```python
from build123d import *

# Parameters (mm, degrees)
BOSS_EXTRUDE1_DEPTH = 34
SKETCH7_W           = 4
SKETCH7_H           = 8
BOSS_EXTRUDE3_DEPTH = 10
SKETCH9_R           = 1.51
CUT_EXTRUDE5_DEPTH  = 48.193431746
FILLET2_R           = 4
SKETCH16_R          = 1.5
CUT_EXTRUDE7_DEPTH  = 30
CHAMFER1_SIZE       = 2


# Some blends are built 0.0001 mm under size
with BuildPart() as part:
    # Sketch1 → Boss-Extrude1 (new body)
    with BuildSketch(Plane(origin=(0, 0, 0), x_dir=(1, 0, 0), z_dir=(0, 1, 0))):
        with BuildLine():
            Line((-7.9, 5.966573556), (-7.9, -5.966573556))
            ThreePointArc((-7.9, -5.966573556), (0, -9.9), (7.9, -5.966573556))
            Line((7.9, -5.966573556), (7.9, 5.966573556))
            ThreePointArc((7.9, 5.966573556), (0, 9.9), (-7.9, 5.966573556))
        make_face()
    extrude(amount=BOSS_EXTRUDE1_DEPTH)

    # Sketch7 → Boss-Extrude3 (add)
    with BuildSketch(Plane(origin=(0, 34, 0), x_dir=(1, 0, 0), z_dir=(0, 1, 0))):
        with Locations((-4, 0)):
            Rectangle(SKETCH7_W, SKETCH7_H)
        with Locations((4, 0)):
            Rectangle(SKETCH7_W, SKETCH7_H)
    extrude(amount=BOSS_EXTRUDE3_DEPTH)

    # Sketch9 → Cut-Extrude5 (cut, through all)
    with BuildSketch(Plane(origin=(6, 0, 0), x_dir=(0, 0, -1), z_dir=(1, 0, 0))):
        with Locations((0, 40)):
            Circle(SKETCH9_R)
    extrude(amount=-CUT_EXTRUDE5_DEPTH, mode=Mode.SUBTRACT)

    # Fillet2
    fillet2_edges = [part.edges().sort_by_distance(p)[0] for p in [
        (4, 44, 4),
        (4, 44, -4),
        (-4, 44, -4),
        (-4, 44, 4),
    ]]
    fillet(fillet2_edges, radius=FILLET2_R - 0.0001)  # a hair under: the kernel refuses the full size

    # Sketch16 → Cut-Extrude7 (cut)
    with BuildSketch(Plane.XZ):
        with Locations(Location((0, 0, 0), (0, 0, 270))):
            Circle(SKETCH16_R)
    extrude(amount=-CUT_EXTRUDE7_DEPTH, mode=Mode.SUBTRACT)

    # Chamfer1
    # the kernel refuses this chamfer: 2 mm, written as the material it adds along each edge
    with BuildSketch(Plane(origin=(-6, 34, -4), x_dir=(0, -0.027495876610585623, -0.9996219169112968), z_dir=(1, 0, 0)), Plane(origin=(2, 34, -4), x_dir=(0, -0.027495876610585623, -0.9996219169112968), z_dir=(1, 0, 0)), Plane(origin=(6, 34, 4), x_dir=(0, -0.027495876610585623, 0.9996219169112968), z_dir=(-1, 0, 0))) as chamfer1_piece_1:
        Polygon((CHAMFER1_SIZE * 0.999621916911, CHAMFER1_SIZE * 0.0274958766106), (-CHAMFER1_SIZE * 0.0274958766106, CHAMFER1_SIZE * 0.999621916911), (0, 0), align=None)
    extrude(amount=4)
    with BuildSketch(Plane(origin=(-6, 34, -4), x_dir=(0, -0.027495876610585623, -0.9996219169112968), z_dir=(1, 0, 0))) as chamfer1_piece_2_section:
        Polygon((CHAMFER1_SIZE * 0.999621916911, CHAMFER1_SIZE * 0.0274958766106), (-CHAMFER1_SIZE * 0.0274958766106, CHAMFER1_SIZE * 0.999621916911), (0, 0), align=None)
    chamfer1_piece_2 = extrude(amount=9.143365976, mode=Mode.PRIVATE)
    chamfer1_piece_2 = split(chamfer1_piece_2, bisect_by=Plane(origin=(2, 34.659587254, -4.659587254), z_dir=(1, 0, 0)), keep=Keep.TOP, mode=Mode.PRIVATE)
    add(chamfer1_piece_2)
    with BuildSketch(Plane(origin=(-6, 34, 4), x_dir=(0.02749587661058651, 0.9996219169112968, 0), z_dir=(0, 0, -1))) as chamfer1_piece_3_section:
        Polygon((CHAMFER1_SIZE * 0.999621916911, -CHAMFER1_SIZE * 0.0274958766106), (-CHAMFER1_SIZE * 0.0274958766106, -CHAMFER1_SIZE * 0.999621916911), (0, 0), align=None)
    chamfer1_piece_3 = extrude(amount=8, mode=Mode.PRIVATE)
    chamfer1_piece_3 = split(chamfer1_piece_3, bisect_by=Plane(origin=(-7.9, 34.66508919, 0), z_dir=(1, 0, 0)), keep=Keep.TOP, mode=Mode.PRIVATE)
    add(chamfer1_piece_3)
    with BuildSketch(Plane(origin=(3.143365976, 34, 4), x_dir=(0, 0.9996219169112968, -0.027495876610586296), z_dir=(-1, 0, 0))) as chamfer1_piece_4_section:
        Polygon((CHAMFER1_SIZE * 0.999621916911, -CHAMFER1_SIZE * 0.0274958766106), (-CHAMFER1_SIZE * 0.0274958766106, -CHAMFER1_SIZE * 0.999621916911), (0, 0), align=None)
    chamfer1_piece_4 = extrude(amount=9.143365976, mode=Mode.PRIVATE)
    chamfer1_piece_4 = split(chamfer1_piece_4, bisect_by=Plane(origin=(2, 34.659587254, 4.659587254), z_dir=(1, 0, 0)), keep=Keep.TOP, mode=Mode.PRIVATE)
    add(chamfer1_piece_4)
    with BuildSketch(Plane(origin=(-2, 34, 4), x_dir=(0, 0.9996219169112968, -0.027495876610586296), z_dir=(-1, 0, 0))) as chamfer1_piece_5:
        Polygon((CHAMFER1_SIZE * 0.999621916911, -CHAMFER1_SIZE * 0.0274958766106), (-CHAMFER1_SIZE * 0.0274958766106, -CHAMFER1_SIZE * 0.999621916911), (0, 0), align=None)
    extrude(amount=4)
    with BuildSketch(Plane(origin=(-3.143365976, 34, -4), x_dir=(0, -0.027495876610585623, -0.9996219169112968), z_dir=(1, 0, 0))) as chamfer1_piece_6_section:
        Polygon((CHAMFER1_SIZE * 0.999621916911, CHAMFER1_SIZE * 0.0274958766106), (-CHAMFER1_SIZE * 0.0274958766106, CHAMFER1_SIZE * 0.999621916911), (0, 0), align=None)
    chamfer1_piece_6 = extrude(amount=9.143365976, mode=Mode.PRIVATE)
    chamfer1_piece_6 = split(chamfer1_piece_6, bisect_by=Plane(origin=(-2, 34.659587254, -4.659587254), z_dir=(-1, 0, 0)), keep=Keep.TOP, mode=Mode.PRIVATE)
    add(chamfer1_piece_6)
    with BuildSketch(Plane(origin=(6, 34, 4), x_dir=(0, -0.027495876610585623, 0.9996219169112968), z_dir=(-1, 0, 0))) as chamfer1_piece_7_section:
        Polygon((CHAMFER1_SIZE * 0.999621916911, CHAMFER1_SIZE * 0.0274958766106), (-CHAMFER1_SIZE * 0.0274958766106, CHAMFER1_SIZE * 0.999621916911), (0, 0), align=None)
    chamfer1_piece_7 = extrude(amount=9.143365976, mode=Mode.PRIVATE)
    chamfer1_piece_7 = split(chamfer1_piece_7, bisect_by=Plane(origin=(-2, 34.659587254, 4.659587254), z_dir=(-1, 0, 0)), keep=Keep.TOP, mode=Mode.PRIVATE)
    add(chamfer1_piece_7)
    with BuildSketch(Plane(origin=(6, 34, -4), x_dir=(0.9996219169112968, -0.027495876610585623, 0), z_dir=(0, 0, 1))) as chamfer1_piece_8_section:
        Polygon((CHAMFER1_SIZE * 0.999621916911, CHAMFER1_SIZE * 0.0274958766106), (-CHAMFER1_SIZE * 0.0274958766106, CHAMFER1_SIZE * 0.999621916911), (0, 0), align=None)
    chamfer1_piece_8 = extrude(amount=8, mode=Mode.PRIVATE)
    chamfer1_piece_8 = split(chamfer1_piece_8, bisect_by=Plane(origin=(7.9, 34.66508919, 0), z_dir=(-1, 0, 0)), keep=Keep.TOP, mode=Mode.PRIVATE)
    add(chamfer1_piece_8)
    with BuildSketch(Plane(origin=(-6, 34, 4), x_dir=(0.02749587661058651, 0.9996219169112968, 0), z_dir=(0, 0, -1))) as chamfer1_piece_9a_section:
        Polygon((CHAMFER1_SIZE * 0.999621916911, -CHAMFER1_SIZE * 0.0274958766106), (-CHAMFER1_SIZE * 0.0274958766106, -CHAMFER1_SIZE * 0.999621916911), (0, 0), align=None)
    chamfer1_piece_9a = extrude(amount=13.143365976, mode=Mode.PRIVATE)
    chamfer1_piece_9a = split(chamfer1_piece_9a, bisect_by=Plane(origin=(-6.579477658, 34.702229701, -4), z_dir=(0, 0, -1)), keep=Keep.TOP, mode=Mode.PRIVATE)
    chamfer1_piece_9a = chamfer1_piece_9a & Plane(origin=(0, 34.702229701, 0), x_dir=(-0.7979797979797981, 0, 0.6026841975828805), z_dir=(0, -1, 0)) * Cylinder(9.9, 35, mode=Mode.PRIVATE)
    chamfer1_piece_9a = split(chamfer1_piece_9a, bisect_by=Plane(origin=(-7.9, 34.702229701, -5.684853753), z_dir=(1, 0, 0)), keep=Keep.TOP, mode=Mode.PRIVATE)
    with BuildSketch(Plane(origin=(-11.143365976, 34, -4), x_dir=(0, -0.027495876610585623, -0.9996219169112968), z_dir=(1, 0, 0))) as chamfer1_piece_9b_section:
        Polygon((CHAMFER1_SIZE * 0.999621916911, CHAMFER1_SIZE * 0.0274958766106), (-CHAMFER1_SIZE * 0.0274958766106, CHAMFER1_SIZE * 0.999621916911), (0, 0), align=None)
    chamfer1_piece_9b = extrude(amount=9.143365976, mode=Mode.PRIVATE)
    chamfer1_piece_9b = split(chamfer1_piece_9b, bisect_by=Plane(origin=(-6, 34.659622918, -4.659519528), z_dir=(-1, 0, 0)), keep=Keep.TOP, mode=Mode.PRIVATE)
    chamfer1_piece_9b = split(chamfer1_piece_9b, bisect_by=Plane(origin=(-7.9, 34.659622918, -4.659519528), z_dir=(1, 0, 0)), keep=Keep.TOP, mode=Mode.PRIVATE)
    chamfer1_piece_9b = chamfer1_piece_9b & Plane(origin=(0, 34.659622918, 0), x_dir=(0.7979797979797981, 0, -0.6026841975828805), z_dir=(0, -1, 0)) * Cylinder(9.9, 27, mode=Mode.PRIVATE)
    chamfer1_piece_9 = chamfer1_piece_9a & chamfer1_piece_9b
    add(chamfer1_piece_9)
    with BuildSketch(Plane(origin=(-6, 34, 9.143365976), x_dir=(0.02749587661058651, 0.9996219169112968, 0), z_dir=(0, 0, -1))) as chamfer1_piece_10a_section:
        Polygon((CHAMFER1_SIZE * 0.999621916911, -CHAMFER1_SIZE * 0.0274958766106), (-CHAMFER1_SIZE * 0.0274958766106, -CHAMFER1_SIZE * 0.999621916911), (0, 0), align=None)
    chamfer1_piece_10a = extrude(amount=13.143365976, mode=Mode.PRIVATE)
    chamfer1_piece_10a = split(chamfer1_piece_10a, bisect_by=Plane(origin=(-6.579477657, 34.702229707, 4), z_dir=(0, 0, 1)), keep=Keep.TOP, mode=Mode.PRIVATE)
    chamfer1_piece_10a = chamfer1_piece_10a & Plane(origin=(0, 34.702229707, 0), x_dir=(-0.7979797979797981, 0, 0.6026841975828805), z_dir=(0, -1, 0)) * Cylinder(9.9, 35, mode=Mode.PRIVATE)
    chamfer1_piece_10a = split(chamfer1_piece_10a, bisect_by=Plane(origin=(-7.9, 34.702229707, 5.684853748), z_dir=(1, 0, 0)), keep=Keep.TOP, mode=Mode.PRIVATE)
    with BuildSketch(Plane(origin=(-2, 34, 4), x_dir=(0, 0.9996219169112968, -0.027495876610586296), z_dir=(-1, 0, 0))) as chamfer1_piece_10b_section:
        Polygon((CHAMFER1_SIZE * 0.999621916911, -CHAMFER1_SIZE * 0.0274958766106), (-CHAMFER1_SIZE * 0.0274958766106, -CHAMFER1_SIZE * 0.999621916911), (0, 0), align=None)
    chamfer1_piece_10b = extrude(amount=9.143365976, mode=Mode.PRIVATE)
    chamfer1_piece_10b = split(chamfer1_piece_10b, bisect_by=Plane(origin=(-6, 34.659622918, 4.659519528), z_dir=(-1, 0, 0)), keep=Keep.TOP, mode=Mode.PRIVATE)
    chamfer1_piece_10b = chamfer1_piece_10b & Plane(origin=(0, 34.659622918, 0), x_dir=(-0.7979797979797981, 0, 0.6026841975828805), z_dir=(0, -1, 0)) * Cylinder(9.9, 27, mode=Mode.PRIVATE)
    chamfer1_piece_10b = split(chamfer1_piece_10b, bisect_by=Plane(origin=(-7.9, 34.659622918, 4.659519528), z_dir=(1, 0, 0)), keep=Keep.TOP, mode=Mode.PRIVATE)
    chamfer1_piece_10 = chamfer1_piece_10a & chamfer1_piece_10b
    add(chamfer1_piece_10)
    with BuildSketch(Plane(origin=(6, 34, -9.143365976), x_dir=(0.9996219169112968, -0.027495876610585623, 0), z_dir=(0, 0, 1))) as chamfer1_piece_11a_section:
        Polygon((CHAMFER1_SIZE * 0.999621916911, CHAMFER1_SIZE * 0.0274958766106), (-CHAMFER1_SIZE * 0.0274958766106, CHAMFER1_SIZE * 0.999621916911), (0, 0), align=None)
    chamfer1_piece_11a = extrude(amount=13.143365976, mode=Mode.PRIVATE)
    chamfer1_piece_11a = chamfer1_piece_11a & Plane(origin=(0, 34.702229706, 0), x_dir=(-0.7979797979797981, 0, 0.6026841975828805), z_dir=(0, -1, 0)) * Cylinder(9.9, 35, mode=Mode.PRIVATE)
    chamfer1_piece_11a = split(chamfer1_piece_11a, bisect_by=Plane(origin=(7.9, 34.702229706, -5.684853749), z_dir=(-1, 0, 0)), keep=Keep.TOP, mode=Mode.PRIVATE)
    chamfer1_piece_11a = split(chamfer1_piece_11a, bisect_by=Plane(origin=(6.579477658, 34.702229706, -4), z_dir=(0, 0, -1)), keep=Keep.TOP, mode=Mode.PRIVATE)
    with BuildSketch(Plane(origin=(2, 34, -4), x_dir=(0, -0.027495876610585623, -0.9996219169112968), z_dir=(1, 0, 0))) as chamfer1_piece_11b_section:
        Polygon((CHAMFER1_SIZE * 0.999621916911, CHAMFER1_SIZE * 0.0274958766106), (-CHAMFER1_SIZE * 0.0274958766106, CHAMFER1_SIZE * 0.999621916911), (0, 0), align=None)
    chamfer1_piece_11b = extrude(amount=9.143365976, mode=Mode.PRIVATE)
    chamfer1_piece_11b = split(chamfer1_piece_11b, bisect_by=Plane(origin=(7.9, 34.659622918, -4.659519528), z_dir=(-1, 0, 0)), keep=Keep.TOP, mode=Mode.PRIVATE)
    chamfer1_piece_11b = chamfer1_piece_11b & Plane(origin=(0, 34.659622918, 0), x_dir=(0.7979797979797981, 0, -0.6026841975828805), z_dir=(0, -1, 0)) * Cylinder(9.9, 27, mode=Mode.PRIVATE)
    chamfer1_piece_11b = split(chamfer1_piece_11b, bisect_by=Plane(origin=(6, 34.659622918, -4.659519528), z_dir=(1, 0, 0)), keep=Keep.TOP, mode=Mode.PRIVATE)
    chamfer1_piece_11 = chamfer1_piece_11a & chamfer1_piece_11b
    add(chamfer1_piece_11)
    with BuildSketch(Plane(origin=(11.143365976, 34, 4), x_dir=(0, -0.027495876610585623, 0.9996219169112968), z_dir=(-1, 0, 0))) as chamfer1_piece_12a_section:
        Polygon((CHAMFER1_SIZE * 0.999621916911, CHAMFER1_SIZE * 0.0274958766106), (-CHAMFER1_SIZE * 0.0274958766106, CHAMFER1_SIZE * 0.999621916911), (0, 0), align=None)
    chamfer1_piece_12a = extrude(amount=9.143365976, mode=Mode.PRIVATE)
    chamfer1_piece_12a = chamfer1_piece_12a & Plane(origin=(0, 34.659622918, 0), x_dir=(-0.7979797979797981, 0, 0.6026841975828805), z_dir=(0, -1, 0)) * Cylinder(9.9, 27, mode=Mode.PRIVATE)
    chamfer1_piece_12a = split(chamfer1_piece_12a, bisect_by=Plane(origin=(7.9, 34.659622918, 4.659519528), z_dir=(-1, 0, 0)), keep=Keep.TOP, mode=Mode.PRIVATE)
    chamfer1_piece_12a = split(chamfer1_piece_12a, bisect_by=Plane(origin=(6, 34.659622918, 4.659519528), z_dir=(1, 0, 0)), keep=Keep.TOP, mode=Mode.PRIVATE)
    with BuildSketch(Plane(origin=(6, 34, -4), x_dir=(0.9996219169112968, -0.027495876610585623, 0), z_dir=(0, 0, 1))) as chamfer1_piece_12b_section:
        Polygon((CHAMFER1_SIZE * 0.999621916911, CHAMFER1_SIZE * 0.0274958766106), (-CHAMFER1_SIZE * 0.0274958766106, CHAMFER1_SIZE * 0.999621916911), (0, 0), align=None)
    chamfer1_piece_12b = extrude(amount=13.143365976, mode=Mode.PRIVATE)
    chamfer1_piece_12b = chamfer1_piece_12b & Plane(origin=(0, 34.702229701, 0), x_dir=(-0.7979797979797981, 0, 0.6026841975828805), z_dir=(0, -1, 0)) * Cylinder(9.9, 35, mode=Mode.PRIVATE)
    chamfer1_piece_12b = split(chamfer1_piece_12b, bisect_by=Plane(origin=(7.9, 34.702229701, 5.684853753), z_dir=(-1, 0, 0)), keep=Keep.TOP, mode=Mode.PRIVATE)
    chamfer1_piece_12b = split(chamfer1_piece_12b, bisect_by=Plane(origin=(6.579477658, 34.702229701, 4), z_dir=(0, 0, 1)), keep=Keep.TOP, mode=Mode.PRIVATE)
    chamfer1_piece_12 = chamfer1_piece_12a & chamfer1_piece_12b
    add(chamfer1_piece_12)


solid = part.part
```
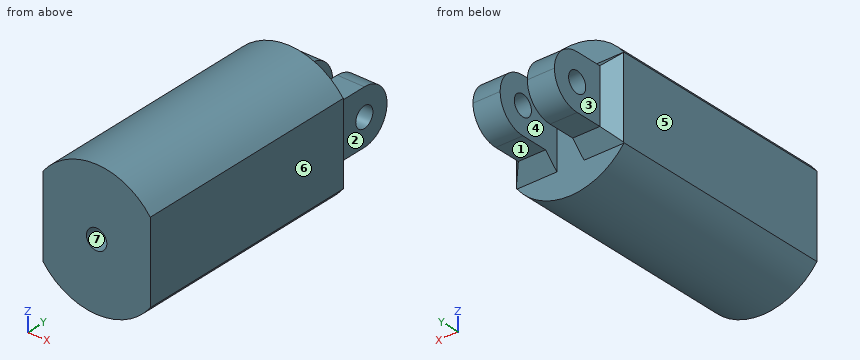
Work out the finished part from the listing and answer in its coordinate system (mm). Face numbers are marked on the shaded views. A direction names the side the tool comes from. Coordinates: 2 decimals unless noted, no trailing zeros. Order: outer loops, then holes, each group sorted by start corner. A loop starts at its lowest first (then second) coordinate and runs counter-clockwise, first axis right, second up. Notation, with made-up numbers: M 45.5,8 L 100.5,8 A29 cw 100.5,46 Z; hole C 31,-17 d2. An arc over 180 degrees is marked long. Use CSV: the item, a comma, the result in double quotes.
1) Determine the mould class of the marked faces 4, 5, 6 and 7 for opening direction X: released by +X, released by -X, zero draft, split by the parting line, or undercut.
Worked out:
face 4,"undercut"
face 5,"released by -X"
face 6,"released by +X"
face 7,"undercut"
2) Consider line 1 (X direction, y = 22, z = 0); line 2 (Y direction, x = 3.65, z = 0); line 3 (X direction, y = 38, z = -2.25). Determine where each line is inside the solid, lowest interval first. Write a range as [from, to].
Worked out:
line 1,"x = [-7.9, -1.5], [1.5, 7.9]"
line 2,"y = [0, 38.49], [41.51, 44]"
line 3,"x = [-6, -2], [2, 6]"
3) Flat-ended cylindrical pins translate along their axes: pin 1 Ø6.5 at (y, z) = (39.5, 0) entering from -X; pin 2 Ø2.5 at (y, z) = (40, 0) entering from -X; pin 3 Ø1.8 at (x, z) = (0, 0) entering from +Y; pin 4 Ø1.2 at (x, y) = (3.5, 38.5) entering from +Z. Find the tip coordinate at first contact, or state that the pin passes through.
Worked out:
pin 1,"stops at x = -6"
pin 2,"passes through"
pin 3,"stops at y = 34"
pin 4,"stops at z = 4"
4) Section D-D on z = 5 is taken. Write down the section's boundary in (x, y).
Worked out:
outline,"M -7.9,0 L 7.9,0 L 7.9,34.1 L 7,35 L 2,35 L 2,34 L -2,34 L -2,35 L -7,35 L -7.9,34.1 Z"
5) Section B-B on y = 26 is taken. Write down the section's boundary in (x, z).
Worked out:
outline,"M -7.9,-5.97 A9.9 ccw 7.9,-5.97 L 7.9,5.97 A9.9 ccw -7.9,5.97 Z; hole C 0,0 d3"
6) For the marked faces 1, 2 and 3, determine the directions among +Z, -Z, +X, -X, +Y, -Y from which every point of the face is accessible in a straight line to the end or side of a thin tool.
Worked out:
face 1,"-Z, +X, -X, +Y"
face 2,"+Z, -Z, +X, +Y"
face 3,"+Z, -Z, -X, +Y"
7) Section A-A on y = 35 is taken. Write down the section's boundary in (x, z).
Worked out:
outline,"M -7,-5 L -2,-5 L -2,5 L -7,5 Z; M 2,-5 L 7,-5 L 7,5 L 2,5 Z"
